Geometry: final body of the model. Coordinates: model frame, mm. Give positions to 0.01 mm unless a question says otherwise; leave off trailing zeros. Loops run counter-clockwise (first coordinate to the right, second up) from the corner with the lowest first, then second, coordinate; pieces in that order, holes last. Notation, with made-up numbers: (71, -17.5) -> (126, -17.5) arc R18 cw to (126, -2.5) -> close; hole circle Ø9 at (37.25, 20.5). An arc over 180 degrees is marked (long way). One line per question, with ' | ' between items. Start each with the question number.
Item 1: Section A-A on x = 108. Return loops of the section in (y, z), then the cut area to 3 significant figures.
Item 2: Section D-D on x = 38. Return loops of the section in (y, z).
Item 3: Material intervals for line 1 along Z through (x, y) = (71.5, 2.55); line 2 along X through (y, z) = (2, -8.5) (3 decimals); line 3 along X through (y, z) = (1.15, -21.25) (3 decimals), sorted ascending. Write a range as [from, to].
Item 4: Pin query (flat end, axial travel): P1, Ø1.2, axis at x = 53, y = 1.5, coming from the -Z side; P2, Ø1.2, axis at y = 1.5, z = -11, coming from the -X side; P3, Ø1.2, axis at x = 100.5, y = 1.5, coming from the +Z side. Return the tip coordinate at first contact, or that it passes through.
Item 5: Section C-C on z = -55. Return loops of the section in (x, y).
Item 6: Section B-B on y = 0.65. Give the number of separate pieces and of enclosed holes in the cut face, then the cut area to 3 significant figures.
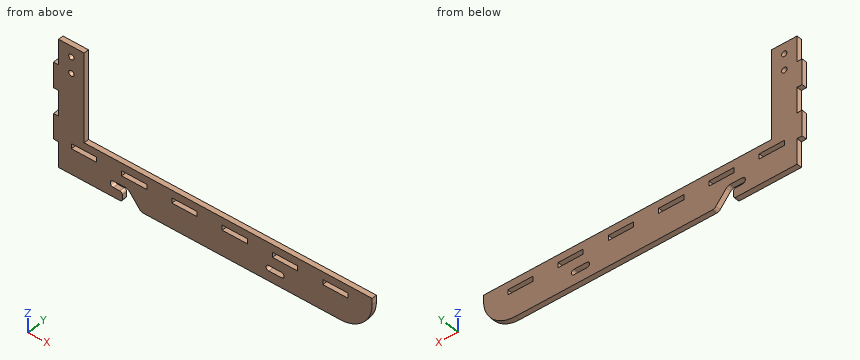
from build123d import *

# Parameters (mm, degrees)
SKETCH1_R           = 2.125
SKETCH1_W           = 19.725
SKETCH1_H           = 4
BOSS_EXTRUDE1_DEPTH = 4


with BuildPart() as part:
    # Sketch1 → Boss-Extrude1 (new body)
    with BuildSketch(Plane(origin=(0, 0, 0), x_dir=(1, 0, 0), z_dir=(0, 1, 0))):
        with BuildLine():
            Line((4, 0), (4, 20))
            Line((4, 20), (0, 20))
            Line((0, 20), (0, 40))
            Line((0, 40), (4, 40))
            Line((4, 40), (4, 60))
            Line((4, 60), (0, 60))
            Line((0, 60), (0, 80))
            Line((0, 80), (4, 80))
            Line((4, 80), (4, 100))
            Line((4, 100), (52, 100))
            ThreePointArc((52, 100), (53.414213562, 99.414213562), (54, 98))
            Line((54, 98), (54, 94.5))
            ThreePointArc((54, 94.5), (53.414213562, 93.085786438), (52, 92.5))
            Line((52, 92.5), (47, 92.5))
            ThreePointArc((47, 92.5), (44.5, 90), (47, 87.5))
            Line((47, 87.5), (56.460109826, 87.5))
            ThreePointArc((56.460109826, 87.5), (58.150582873, 87.874768852), (59.524287598, 88.928849561))
            Line((59.524287598, 88.928849561), (67.615138708, 98.571150439))
            ThreePointArc((67.615138708, 98.571150439), (68.988843434, 99.625231148), (70.679316481, 100))
            Line((70.679316481, 100), (225, 100))
            ThreePointArc((225, 100), (242.67766953, 92.67766953), (250, 75))
            Line((250, 75), (250, 70))
            Line((250, 70), (24, 70))
            Line((24, 70), (24, 0))
            Line((24, 0), (4, 0))
        make_face()
        with Locations((14, 8.5)):
            Circle(SKETCH1_R, mode=Mode.SUBTRACT)
        with Locations((14, 21.25)):
            Circle(SKETCH1_R, mode=Mode.SUBTRACT)
        with Locations((63.3125, 78)):
            Rectangle(SKETCH1_W, SKETCH1_H, mode=Mode.SUBTRACT)
        with Locations((23.8625, 78)):
            Rectangle(SKETCH1_W, SKETCH1_H, mode=Mode.SUBTRACT)
        with Locations((102.7625, 78)):
            Rectangle(SKETCH1_W, SKETCH1_H, mode=Mode.SUBTRACT)
        with Locations((142.2125, 78)):
            Rectangle(SKETCH1_W, SKETCH1_H, mode=Mode.SUBTRACT)
        with Locations((181.6625, 78)):
            Rectangle(SKETCH1_W, SKETCH1_H, mode=Mode.SUBTRACT)
        with Locations((221.1125, 78)):
            Rectangle(SKETCH1_W, SKETCH1_H, mode=Mode.SUBTRACT)
        with BuildLine():
            Line((168.885, 92.125), (178.885, 92.125))
            ThreePointArc((178.885, 92.125), (181.01, 90), (178.885, 87.875))
            Line((178.885, 87.875), (168.885, 87.875))
            ThreePointArc((168.885, 87.875), (166.76, 90), (168.885, 92.125))
        make_face(mode=Mode.SUBTRACT)
    extrude(amount=BOSS_EXTRUDE1_DEPTH)


solid = part.part
Result sheet:
1) outline: (0, -100) -> (4, -100) -> (4, -80) -> (0, -80) -> close; (0, -76) -> (4, -76) -> (4, -70) -> (0, -70) -> close | area: 104 mm²
2) outline: (0, -100) -> (4, -100) -> (4, -70) -> (0, -70) -> close
3) line 1: z = [-100, -80], [-76, -70] | line 2: x = [4, 11.875], [16.125, 24] | line 3: x = [0, 11.875], [16.125, 24]
4) P1: stops at z = -99.96 | P2: stops at x = 4 | P3: stops at z = -70
5) outline: (4, 0) -> (24, 0) -> (24, 4) -> (4, 4) -> close
6) separate pieces: 1 | enclosed holes: 9 | area: 8,080 mm²
